Check sheet for the modelled part. Datum: model origin and axes. Units: mm. A direction names the side the tool comes from. Round coordinates to 2 decimals unless told otherwise and drop trailing zeros. Order: outer loops, then holes, each group sorted by start corner. A loop starts at its lowest first (then second) coordinate and runs counter-clockwise, first axis right, second up. Notation, with made-up numbers: (46, -7.5) -> (61, -7.5) arc R19 cw to (61, 16.5) -> close; hole circle Ø2 at (-10.75, -1.75). An arc over 180 degrees is marked (long way). Answer in a Markdown table with one row per item.
from build123d import *

# Parameters (mm, degrees)
BOSS_EXTRUDE1_START    = -34.925
SKETCH1_W              = 82.55
SKETCH1_H              = 81.407
BOSS_EXTRUDE1_DEPTH    = 3.175
SKETCH3_W              = 82.55
SKETCH3_H              = 3.175
BOSS_EXTRUDE2_DEPTH    = 50.8
F_10_CLEARANCE_HOLE2_D = 5.334
CHAMFER1_SIZE          = 3.175
FILLET2_R              = 3.937
SKETCH9_R              = 3.429
CUT_EXTRUDE2_DEPTH     = 54.975
SKETCH10_W             = 82.55
SKETCH10_H             = 24.638
CUT_EXTRUDE3_DEPTH     = 82.407


with BuildPart() as part:
    # Sketch1 → Boss-Extrude1 (new body)
    with BuildSketch(Plane(origin=(0, 0, 0), x_dir=(1, 0, 0), z_dir=(0, 1, 0)).offset(BOSS_EXTRUDE1_START)):
        Rectangle(SKETCH1_W, SKETCH1_H)
    extrude(amount=BOSS_EXTRUDE1_DEPTH)

    # Sketch3 → Boss-Extrude2 (add)
    with BuildSketch(Plane(origin=(0, -31.75, 0), x_dir=(1, 0, 0), z_dir=(0, 1, 0))):
        with Locations((0, -39.116)):
            Rectangle(SKETCH3_W, SKETCH3_H)
    extrude(amount=BOSS_EXTRUDE2_DEPTH)

    # #10 Clearance Hole2 (through all)
    with Locations(Plane(origin=(0, 0, -40.7035), x_dir=(-1, 0, 0), z_dir=(0, 0, -1))):
        with Locations((22.225, 7.112), (9.525, 7.112), (-3.175, 7.112), (-15.875, 7.112), (-28.575, 7.112), (22.225, -18.288), (9.525, -18.288), (-3.175, -18.288), (-15.875, -18.288), (-28.575, -18.288), (34.925, 7.112), (34.925, -18.288), (-41.275, 7.112), (-41.275, -18.288)):
            Hole(F_10_CLEARANCE_HOLE2_D / 2)

    # Chamfer1
    chamfer1_edges = [part.edges().sort_by_distance(p)[0] for p in [
        (-41.275, 19.05, 39.116),
    ]]
    chamfer(chamfer1_edges, length=CHAMFER1_SIZE)

    # Fillet2
    fillet2_edges = [part.edges().sort_by_distance(p)[0] for p in [
        (0, -34.925, 40.7035),
    ]]
    fillet(fillet2_edges, radius=FILLET2_R)

    # Sketch9 → Cut-Extrude2 (cut, through all)
    with BuildSketch(Plane.XZ.offset(34.925)):
        with Locations((28.575, 24.8285)):
            Circle(SKETCH9_R)
        with Locations((28.575, -0.5715)):
            Circle(SKETCH9_R)
        with Locations((28.575, -25.9715)):
            Circle(SKETCH9_R)
        Polygon((-41.275, 37.5285), (15.875, -40.7035), (-41.275, -40.7035), align=None)
    extrude(amount=-CUT_EXTRUDE2_DEPTH, mode=Mode.SUBTRACT)

    # Sketch10 → Cut-Extrude3 (cut, through all)
    with BuildSketch(Plane.XY.offset(40.7035)):
        with Locations((0, 6.731)):
            Rectangle(SKETCH10_W, SKETCH10_H)
    extrude(amount=-CUT_EXTRUDE3_DEPTH, mode=Mode.SUBTRACT)


solid = part.part
Item 1: Cross-section at B-B (x = 28). State how many separate pieces and enclosed holes the cut face has, and give its area (3 significant figures).
Result sheet:
| item | result |
|---|---|
| separate pieces | 5 |
| enclosed holes | 0 |
| area | 257 mm^2 |
Item 2: Depth check by flat-ended pin: P1, Ø8, axis at x = -7.5, y = -19.5, coming from the -Z side; P2, Ø5, axis at x = 3.175, y = -18.288, coming from the -Z side; P3, Ø4, axis at x = 1, z = -15, coming from the +Y side. Enter the tip coordinate at first touch or a pass-through.
Result sheet:
| item | result |
|---|---|
| P1 | stops at z = 37.53 |
| P2 | passes through |
| P3 | stops at y = -31.75 |
Item 3: Mould release check, pull along Y, two halves, no side actions. Record for faces 1 (the flat face through (-13.1, -33.36, -1.04)), 2 (the cylindrical face through (38.61, -18.23, 39.14)), 3 (the cylindrical face through (-19.76, -19.31, 39.14)), 4 (the flat face through (9, -34.925, 6)): pulls with the +Y half, pulls with the -Y half, needs draft (parallel to the pull), parting line crosses it, or undercut.
Result sheet:
| item | result |
|---|---|
| face 1 | needs draft |
| face 2 | undercut |
| face 3 | undercut |
| face 4 | pulls with the -Y half |
Item 4: Cross-section at C-C (z = 0.5). Record the boundary of the cut face in (x, y) (3 decimals), and give its area (3 significant figures).
Result sheet:
| item | result |
|---|---|
| outline | (-14.225, -34.925) -> (25.318, -34.925) -> (25.318, -31.75) -> (-14.225, -31.75) -> close; (31.832, -34.925) -> (41.275, -34.925) -> (41.275, -31.75) -> (31.832, -31.75) -> close |
| area | 156 mm^2 |
Item 5: Cross-section at A-A (y = -16.75). Record the boundary of the cut face in (x, z) (1 decimal), and give its area (3 significant figures).
Result sheet:
| item | result |
|---|---|
| outline | (-41.3, 37.5) -> (-37.1, 37.5) -> (-37.1, 40.7) -> (-41.3, 40.7) -> close; (-32.7, 37.5) -> (-24.4, 37.5) -> (-24.4, 40.7) -> (-32.7, 40.7) -> close; (-20, 37.5) -> (-11.7, 37.5) -> (-11.7, 40.7) -> (-20, 40.7) -> close; (-7.3, 37.5) -> (1, 37.5) -> (1, 40.7) -> (-7.3, 40.7) -> close; (5.4, 37.5) -> (13.7, 37.5) -> (13.7, 40.7) -> (5.4, 40.7) -> close; (18.1, 37.5) -> (26.4, 37.5) -> (26.4, 40.7) -> (18.1, 40.7) -> close; (30.8, 37.5) -> (39.1, 37.5) -> (39.1, 40.7) -> (30.8, 40.7) -> close |
| area | 172 mm^2 |
Item 6: Set-up check for faces 5 (the cylindrical face through (30.16, -33.36, -29.01)), 6 (the flat face through (9, -31.75, 7)): record each of +Z, -Z, +X, -X, +Y, -Y from which the full face is reachable in a straight line by a thin tool's end or side.
Result sheet:
| item | result |
|---|---|
| face 5 | +Y, -Y |
| face 6 | -Z, +X, -X, +Y |
Item 7: Scan lines: line 1 (Y direction, x = 30, z = -13) (3 decimals); line 2 (Z direction, x = 26.5, y = -16.5); line 3 (X direction, y = -32, z = 32.5) (3 decimals). Record each from-to range of solid material in increasing order. Write a range as [from, to].
Result sheet:
| item | result |
|---|---|
| line 1 | y = [-34.925, -31.75] |
| line 2 | z = [37.53, 40.7] |
| line 3 | x = [-37.602, 41.275] |
Item 8: Cross-section at D-D (y = -28.5). Record the boundary of the cut face in (x, z) (1 decimal), and give its area (3 significant figures).
Result sheet:
| item | result |
|---|---|
| outline | (-41.3, 37.5) -> (41.3, 37.5) -> (41.3, 40.7) -> (-41.3, 40.7) -> close |
| area | 262 mm^2 |
